Geometry check sheet. Reference: the model listing, model coordinates, mm. A direction names the side the tool comes from. Give positions to 0.01 mm unless a question says otherwise; leave off trailing zeros. Loops run counter-clockwise (first coordinate to the right, second up) from the corner with the lowest first, then second, coordinate; pieces in that order, holes last. Notation, with made-up numbers: (48.25, -30) -> (73.25, -30) arc R20 cw to (73.25, -22) -> close; hole circle Ø9 at (44.5, 46.25). An arc over 180 degrees is marked (long way). Write item = value, one per line. Start each with the question number.
```python
from build123d import *

# Parameters (mm, degrees)
SKETCH1_R           = 1.5
BOSS_EXTRUDE1_DEPTH = 4
CUT_EXTRUDE2_DEPTH  = 5
CIRPATTERN1_COUNT   = 12
SKETCH3_W           = 7.863082298
SKETCH3_H           = 5
BOSS_EXTRUDE2_DEPTH = 4
SKETCH4_R           = 2.5
CUT_EXTRUDE3_DEPTH  = 5


with BuildPart() as part:
    # Sketch1 → Boss-Extrude1 (new body)
    with BuildSketch(Plane.XY):
        with BuildLine():
            Line((-18, 2.5), (12.545643943, 2.5))
            ThreePointArc((12.545643943, 2.5), (24, 0), (12.545643943, -2.5))
            Line((12.545643943, -2.5), (-18, -2.5))
            ThreePointArc((-18, -2.5), (-20.5, 0), (-18, 2.5))
        make_face()
        with Locations((-18, 0)):
            Circle(SKETCH1_R, mode=Mode.SUBTRACT)
    extrude(amount=BOSS_EXTRUDE1_DEPTH)

    # Sketch2 → Cut-Extrude2 (cut, through all)
    with BuildSketch(Plane.XY.offset(4)):
        with BuildLine():
            Line((20.008070513, 4.695554958), (19.882890915, 4.479152397))
            ThreePointArc((19.882890915, 4.479152397), (19.821496871, 4.016588638), (20.105, 3.64596695))
            ThreePointArc((20.105, 3.64596695), (20.567719361, 3.585756883), (20.937614306, 3.870207564))
            Line((20.937614306, 3.870207564), (21.062434622, 4.086817556))
            ThreePointArc((21.062434622, 4.086817556), (21.614093727, 4.455903836), (22.242640687, 4.242640687))
            ThreePointArc((22.242640687, 4.242640687), (21.17938524, 5.506856773), (19.552914271, 5.795554958))
            ThreePointArc((19.552914271, 5.795554958), (20.051879055, 5.357848898), (20.008070513, 4.695554958))
        make_face()
    cut_extrude2 = extrude(amount=-CUT_EXTRUDE2_DEPTH, mode=Mode.SUBTRACT)

    # CirPattern1: Cut-Extrude2 ×12 about axis
    cirpattern1_axis = Axis((18, 0, 0), (0, 0, 1))
    for i in range(1, CIRPATTERN1_COUNT):
        add(cut_extrude2.rotate(cirpattern1_axis, i * 360 / CIRPATTERN1_COUNT), mode=Mode.SUBTRACT)

    # Sketch3 → Boss-Extrude2 (add)
    with BuildSketch(Plane.XY.offset(4)):
        with Locations((12.029323846, 0)):
            Rectangle(SKETCH3_W, SKETCH3_H)
    extrude(amount=-BOSS_EXTRUDE2_DEPTH)

    # Sketch4 → Cut-Extrude3 (cut, through all)
    with BuildSketch(Plane.XY.offset(4)):
        with Locations((18, 0)):
            Circle(SKETCH4_R)
    extrude(amount=-CUT_EXTRUDE3_DEPTH, mode=Mode.SUBTRACT)


solid = part.part
```
1) Thickness scan on line 1 (Y direction, x = -18, z = 2.45); line 2 (X direction, y = -1.25, z = 0.25); line 3 (X direction, y = -0.75, z = 1.05). Record the ranges inside material, lowest first.
2) Section check A-A (x = 19). Enter the section's corners in (y, z), plus the area to 3 significant figures.
3) Tool access check on faces 1 (the cylindrical face through (15.426, 3.588, 2.028)), 2 (the cylindrical face through (22.02, -1.82, 2.03)). Record the directions out of +Z, -Z, +X, -X, +Y, -Y that give a thin tool (end or side, any length) a straight path to the whole face; none if there is none.
4) Section check C-C (x = -17). Enter the section's corners in (y, z), plus the area to 3 significant figures.
5) Section check D-D (x = -9.5). Enter the section's corners in (y, z), plus the area to 3 significant figures.
6) Section check B-B (z = 0.4). Give the number of separate pieces and of enclosed holes in the cut face, plus the area to 3 significant figures.
7) Draft check along X on faces 3 (the cylindrical face through (-20.5, -0.1, 2)), 4 (the cylindrical face through (16.18, -4.02, 2.03)), 5 (the cylindrical face through (16.177, 4.01, 2.028)), 6 (the flat face through (-2, -2.5, 2)). Enter one of: released by +X, released by -X, zero draft, split by the parting line, or undercut.
8) Depth check by flat-ended pin: pin 1 Ø5 at (x, y) = (5.5, 2.5) entering from -Z; pin 2 Ø1.2 at (x, z) = (5, 2) entering from -Y. Enter the tip coordinate at first touch or a pass-through.
Check result:
q1.line_1 = -2.5 to -1.5, 1.5 to 2.5
q1.line_2 = -20.17 to -18.83, -17.17 to 15.83, 20.17 to 23.81
q1.line_3 = -20.38 to -19.3, -16.7 to 15.62, 20.38 to 23.51
q2.outline = (-5.73, 0) -> (-2.29, 0) -> (-2.29, 4) -> (-5.73, 4) -> close; (2.29, 0) -> (5.73, 0) -> (5.73, 4) -> (2.29, 4) -> close
q2.area = 27.5 mm2
q3.face_1 = +Z, -Z, +Y
q3.face_2 = +Z, -Z
q4.outline = (-2.5, 0) -> (-1.12, 0) -> (-1.12, 4) -> (-2.5, 4) -> close; (1.12, 0) -> (2.5, 0) -> (2.5, 4) -> (1.12, 4) -> close
q4.area = 11.1 mm2
q5.outline = (-2.5, 0) -> (2.5, 0) -> (2.5, 4) -> (-2.5, 4) -> close
q5.area = 20.0 mm2
q6.separate_pieces = 1
q6.enclosed_holes = 2
q6.area = 223 mm2
q7.face_3 = released by -X
q7.face_4 = undercut
q7.face_5 = undercut
q7.face_6 = zero draft
q8.pin_1 = 0
q8.pin_2 = -2.5
